Design review of the part built by this model. Coordinates are the model's own, in mm. A direction names the side the tool comes from. Round coordinates to 2 decimals unless told otherwise and drop trailing zeros. Loops run counter-clockwise (first coordinate to the right, second up) from the corner with the lowest first, then second, coordinate; pieces in that order, holes last. Notation, with made-up numbers: (85, 85.5) -> (98, 85.5) arc R22 cw to (98, 112.5) -> close; hole circle Ø4 at (18, -39.75). An arc over 180 degrees is marked (long way). Write each question's results on one line, items separated by ' | '. Start each with the question number.
from build123d import *

# Parameters (mm, degrees)
SKETCH_2_W                       = 89.1
SKETCH_2_H                       = 1.5
SM_BASE_FLANGE_1_DEPTH           = 152
SM_EDGE_FLANGE_1_STRIP_W         = 7.4732
SM_EDGE_FLANGE_1_STRIP_H         = 1.5
SM_EDGE_FLANGE_1_STRIP_CUT_DEPTH = 152
SM_EDGE_FLANGE_1_DEPTH           = 152
SM_EDGE_FLANGE_2_STRIP_W         = 7.4732
SM_EDGE_FLANGE_2_STRIP_H         = 1.5
SM_EDGE_FLANGE_2_STRIP_CUT_DEPTH = 152
SM_EDGE_FLANGE_2_DEPTH           = 152
SKETCH_13_W                      = 16.114616681
SKETCH_13_H                      = 12.6
SKETCH_13_W_2                    = 14.895249376
CUT_EXTRUDE_1_DEPTH              = 177.473255764
SM_EDGE_FLANGE_3_STRIP_W         = 7.4732
SM_EDGE_FLANGE_3_STRIP_H         = 1.5
SM_EDGE_FLANGE_3_STRIP_CUT_DEPTH = 84.6268
SM_EDGE_FLANGE_3_DEPTH           = 84.6268
SKETCH_17_R                      = 2.25
CUT_EXTRUDE_2_DEPTH              = 10
SKETCH_18_R                      = 2.25
CUT_EXTRUDE_3_DEPTH              = 10
HOLE_WIZARD_M4_1_D               = 3.3
HOLE_WIZARD_M4_1_DEPTH           = 10.1
HOLE_WIZARD_M4_1_TIP             = 0.991420021


# Sheet-metal steps are written as plain solids
with BuildPart() as part:
    # Sketch 2 → 基体-法兰1 (new body)
    with BuildSketch(Plane.XY):
        with Locations((44.55, -0.75)):
            Rectangle(SKETCH_2_W, SKETCH_2_H)
    extrude(amount=SM_BASE_FLANGE_1_DEPTH)

    # 边线-法兰1 strip (across the edge) → 边线-法兰1 strip cut (cut)
    with BuildSketch(Plane.XY):
        with Locations((-1.5, -0.75)):
            Rectangle(SM_EDGE_FLANGE_1_STRIP_W, SM_EDGE_FLANGE_1_STRIP_H)
    extrude(amount=SM_EDGE_FLANGE_1_STRIP_CUT_DEPTH, mode=Mode.SUBTRACT)

    # 边线-法兰1 section (across the edge) → 边线-法兰1 (add)
    with BuildSketch(Plane.XY):
        with BuildLine():
            Line((0, 0.7366), (0, 8.5))
            Line((0, 8.5), (1.5, 8.5))
            Line((1.5, 8.5), (1.5, 0.7366))
            ThreePointArc((1.5, 0.7366), (1.715745145, 0.215745145), (2.2366, 0))
            Line((2.2366, 0), (2.2366, -1.5))
            ThreePointArc((2.2366, -1.5), (0.655084973, -0.844915027), (0, 0.7366))
        make_face()
    extrude(amount=SM_EDGE_FLANGE_1_DEPTH)

    # 边线-法兰2 strip (across the edge) → 边线-法兰2 strip cut (cut)
    with BuildSketch(Plane(origin=(89.1, 0, 152), x_dir=(-1, 0, 0), z_dir=(0, 0, -1))):
        with Locations((-1.5, -0.75)):
            Rectangle(SM_EDGE_FLANGE_2_STRIP_W, SM_EDGE_FLANGE_2_STRIP_H)
    extrude(amount=SM_EDGE_FLANGE_2_STRIP_CUT_DEPTH, mode=Mode.SUBTRACT)

    # 边线-法兰2 section (across the edge) → 边线-法兰2 (add)
    with BuildSketch(Plane(origin=(89.1, 0, 152), x_dir=(-1, 0, 0), z_dir=(0, 0, -1))):
        with BuildLine():
            Line((0, 0.7366), (0, 8.5))
            Line((0, 8.5), (1.5, 8.5))
            Line((1.5, 8.5), (1.5, 0.7366))
            ThreePointArc((1.5, 0.7366), (1.715745145, 0.215745145), (2.2366, 0))
            Line((2.2366, 0), (2.2366, -1.5))
            ThreePointArc((2.2366, -1.5), (0.655084973, -0.844915027), (0, 0.7366))
        make_face()
    extrude(amount=SM_EDGE_FLANGE_2_DEPTH)

    # 草图13 → 切除-拉伸1 (cut, through all)
    with BuildSketch(Plane.XZ.offset(1.5)):
        with Locations((-5.82070834, 145.7)):
            Rectangle(SKETCH_13_W, SKETCH_13_H)
        with Locations((94.311024688, 145.7)):
            Rectangle(SKETCH_13_W_2, SKETCH_13_H)
    extrude(amount=-CUT_EXTRUDE_1_DEPTH, mode=Mode.SUBTRACT)

    # 边线-法兰3 strip (across the edge) → 边线-法兰3 strip cut (cut)
    with BuildSketch(Plane(origin=(86.8634, -1.5, 152), x_dir=(0, 0, -1), z_dir=(-1, 0, 0))):
        with Locations((-1.5, -0.75)):
            Rectangle(SM_EDGE_FLANGE_3_STRIP_W, SM_EDGE_FLANGE_3_STRIP_H)
    extrude(amount=SM_EDGE_FLANGE_3_STRIP_CUT_DEPTH, mode=Mode.SUBTRACT)

    # 边线-法兰3 section (across the edge) → 边线-法兰3 (add)
    with BuildSketch(Plane(origin=(86.8634, -1.5, 152), x_dir=(0, 0, -1), z_dir=(-1, 0, 0))):
        with BuildLine():
            Line((0, 0.7366), (0, 8.5))
            Line((0, 8.5), (1.5, 8.5))
            Line((1.5, 8.5), (1.5, 0.7366))
            ThreePointArc((1.5, 0.7366), (1.715745145, 0.215745145), (2.2366, 0))
            Line((2.2366, 0), (2.2366, -1.5))
            ThreePointArc((2.2366, -1.5), (0.655084973, -0.844915027), (0, 0.7366))
        make_face()
    extrude(amount=SM_EDGE_FLANGE_3_DEPTH)

    # 草图17 → 切除-拉伸2 (cut)
    with BuildSketch(Plane.XY.offset(152)):
        with Locations((80.55, -6)):
            Circle(SKETCH_17_R)
        with Locations(Location((8.55, -6, 0), (0, 0, 270))):
            Circle(SKETCH_17_R)
    extrude(amount=-CUT_EXTRUDE_2_DEPTH, mode=Mode.SUBTRACT)

    # 草图18 → 切除-拉伸3 (cut)
    with BuildSketch(Plane.XZ.offset(1.5)):
        with Locations(Location((17.05, 145.5, 0), (0, 0, 270))):
            Circle(SKETCH_18_R)
        with Locations(Location((72.05, 145.5, 0), (0, 0, 90))):
            Circle(SKETCH_18_R)
    extrude(amount=-CUT_EXTRUDE_3_DEPTH, mode=Mode.SUBTRACT)

    # M4 螺纹孔1
    with Locations(Plane(origin=(89.1, 0, 0), x_dir=(0, 0, -1), z_dir=(1, 0, 0))):
        with Locations((-30, 4.5)):
            Hole(HOLE_WIZARD_M4_1_D / 2, depth=HOLE_WIZARD_M4_1_DEPTH)
            with Locations((0, 0, -(HOLE_WIZARD_M4_1_DEPTH + HOLE_WIZARD_M4_1_TIP / 2))):  # 118° drill point
                Cone(0, HOLE_WIZARD_M4_1_D / 2, HOLE_WIZARD_M4_1_TIP, mode=Mode.SUBTRACT)


solid = part.part
1) Take a section at D-D (z = 145.5). Write out the cut boundary in (x, y).
2) For faces 4 (the face through (45, -6, 150.5)), 5 (the face through (1.5, 5, 69)), 6 (the face through (88.34, 3.5, 28.69)), 7 (the face through (2.237, -1, 148)), list the 3-axis set-ups (+Z, -Z, +X, -X, +Y, -Y) from which the entire face can be reached by the end or side of a thin tool; tool diameter is ignored.
3) Take a section at C-C (x = 72.05). Write out the cut boundary in (y, z).
4) To check wall thickness, follow line 1 (X direction, y = -0.5, z = 145.5); line 2 (X direction, y = 7, z = 63.5); line 3 (Y direction, x = 21, z = 39.5). State the ranges of each line that lie inside material, in increasing order. Write a range as from..to.
5) The part is to be moulded in two halves that separate along Y. For faces 1 (the face through (44, 0, 74)), 2 (the face through (87.6, 5, 71)), 3 (the face through (82.63, -6.86, 151.26)), say which applies: +Y half, -Y half, draft (parallel to the pull), parting line (faces both ways), or undercut.
6) Take a section at A-A (y = -6). Write out the cut boundary in (x, z), plus the area to 3 significant figures.
7) Insertion check: pin 1 (2 mm diameter, centred on x = 25.5, z = 25.5, fed in from +Y); pin 2 (2.5 mm diameter, centred on x = 80.55, y = -6, fed in from +Z); pin 3 (4 mm diameter, centred on y = -2.5, z = 126.5, fed in from -X); pin 4 (1 mm diameter, centred on x = 65.5, z = 57.5, fed in from -Y). Each pin has a flat end and moves straight along its axis. Give the tip position at first contact, or say it passes through.
8) Take a section at B-B (z = 30). Write out the cut boundary in (x, y).
Geometry check:
1) outline: (2.24, -1.5) -> (14.8, -1.5) -> (14.8, 0) -> (2.24, 0) -> close; (19.3, -1.5) -> (69.8, -1.5) -> (69.8, 0) -> (19.3, 0) -> close; (74.3, -1.5) -> (86.86, -1.5) -> (86.86, 0) -> (74.3, 0) -> close
2) face 4: -Z, +X, -X, -Y | face 5: +Z, -Z, +Y | face 6: +X | face 7: +Z, -X, +Y, -Y
3) outline: (-10, 150.5) -> (-2.24, 150.5) arc R0.74 cw to (-1.5, 149.76) -> (-1.5, 147.75) -> (0, 147.75) -> (0, 149.76) arc R2.24 ccw to (-2.24, 152) -> (-10, 152) -> close; (-1.5, 0) -> (0, 0) -> (0, 143.25) -> (-1.5, 143.25) -> close
4) line 1: x = 2.24..14.8, 19.3..69.8, 74.3..86.86 | line 2: x = 0..1.5, 87.6..89.1 | line 3: y = -1.5..0
5) face 1: +Y half | face 2: draft | face 3: undercut
6) outline: (2.24, 150.5) -> (6.3, 150.5) -> (6.3, 152) -> (2.24, 152) -> close; (10.8, 150.5) -> (78.3, 150.5) -> (78.3, 152) -> (10.8, 152) -> close; (82.8, 150.5) -> (86.86, 150.5) -> (86.86, 152) -> (82.8, 152) -> close | area: 113 mm^2
7) pin 1: stops at y = 0 | pin 2: passes through | pin 3: stops at x = 0.37 | pin 4: stops at y = -1.5
8) outline: (0, 0.74) arc R2.24 ccw to (2.24, -1.5) -> (86.86, -1.5) arc R2.24 ccw to (89.1, 0.74) -> (89.1, 2.85) -> (87.6, 2.85) -> (87.6, 0.74) arc R0.74 cw to (86.86, 0) -> (2.24, 0) arc R0.74 cw to (1.5, 0.74) -> (1.5, 8.5) -> (0, 8.5) -> close; (87.6, 6.15) -> (89.1, 6.15) -> (89.1, 8.5) -> (87.6, 8.5) -> close
